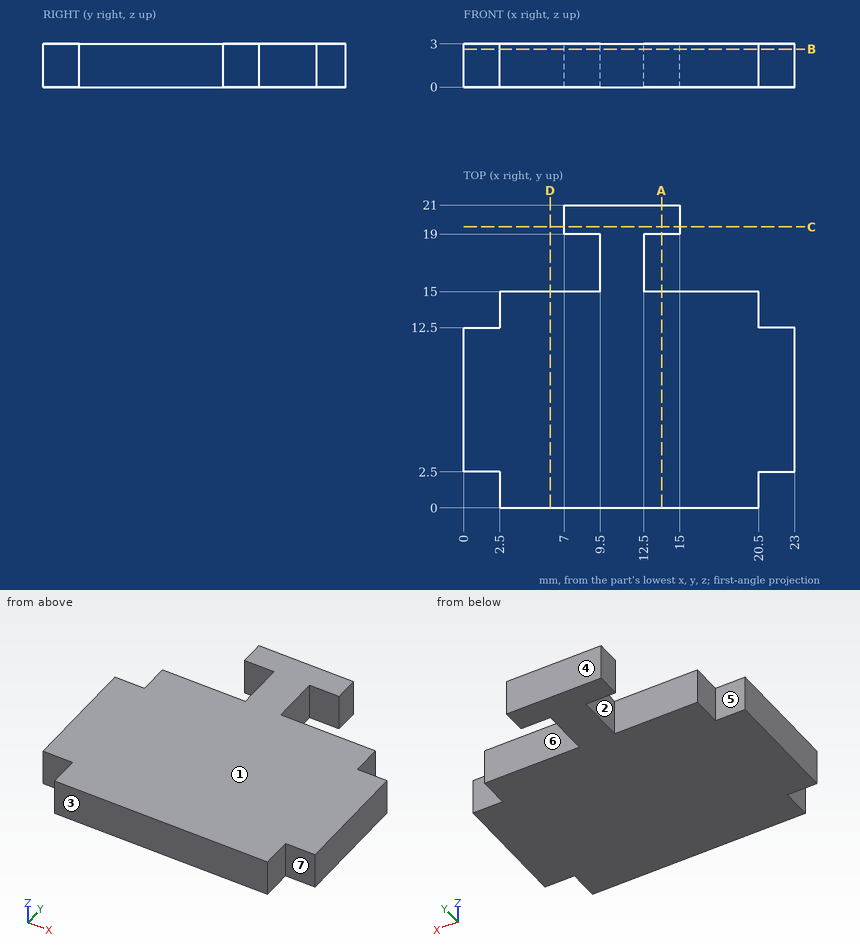
Source: three-view drawing plus pictorial views. Frame: mm from the lowest corner of the part. A direction names the side the tool comes from. Round coordinates to 2 decimals unless told otherwise and drop trailing zeros. Loops run counter-clockwise (first coordinate to the right, second up) from the corner with the lowest first, then second, coordinate; pieces in that order, holes last. Notation, with made-up numbers: M 59,72.25 L 64,72.25 A24 cw 64,87.25 Z; hole C 60.25,20 d1. An arc over 180 degrees is marked long. Answer as CSV lines item,"result". Start each with the question number.
(1) Section A-A, the plane x = 13.75. Output: boundary loops of the cut face in (y, z).
(2) Section D-D, the plane x = 6. Output: boundary loops of the cut face in (y, z), plus the area to 3 significant figures.
(3) First-contact query: pin 1 (1 mm diameter, centred on y = 20, z = 2, fed in from +X); pin 2 (0.8 mm diameter, centred on y = 13.5, z = 1.5, fed in from +X); pin 3 (1.5 mm diameter, centred on y = 17.5, z = 1, fed in from -X). Flat tips, straight axial feed; report the tip coordinate or a pass-through.
(4) Section C-C, the plane y = 19.5. Output: boundary loops of the cut face in (x, z), plus the area to 3 significant figures.
(5) Line query: line 1 (Y direction, x = 9, z = 1.7); line 2 (Y direction, x = 6.75, z = 2.2); line 3 (X direction, y = 17, z = 0.25). Output: solid intervals per line, ascending. Write a range as [from, to].
(6) Section B-B, the plane z = 2.65. Output: boundary loops of the cut face in (x, y), plus the area to 3 significant figures.
(7) Reachability of the marked faces 5, 6 and 7 from +Z, -Z, +X, -X, +Y, -Y: full face, straight path, thin tool, end or side. Return the list, or none.
(8) Draft query along Y for the marked faces 1, 2, 3 and 4. Return one class per face: released by +Y, released by -Y, zero draft, split by the parting line, or undercut.
Values found:
1,outline,"M 0,0 L 15,0 L 15,3 L 0,3 Z; M 19,0 L 21,0 L 21,3 L 19,3 Z"
2,outline,"M 0,0 L 15,0 L 15,3 L 0,3 Z"
2,area,"45.0 mm²"
3,pin 1,"stops at x = 15"
3,pin 2,"stops at x = 20.5"
3,pin 3,"stops at x = 9.5"
4,outline,"M 7,0 L 15,0 L 15,3 L 7,3 Z"
4,area,"24.0 mm²"
5,line 1,"y = [0, 15], [19, 21]"
5,line 2,"y = [0, 15]"
5,line 3,"x = [9.5, 12.5]"
6,outline,"M 0,2.5 L 2.5,2.5 L 2.5,0 L 20.5,0 L 20.5,2.5 L 23,2.5 L 23,12.5 L 20.5,12.5 L 20.5,15 L 12.5,15 L 12.5,19 L 15,19 L 15,21 L 7,21 L 7,19 L 9.5,19 L 9.5,15 L 2.5,15 L 2.5,12.5 L 0,12.5 Z"
6,area,"348 mm²"
7,face 5,"+Z, -Z, -X, +Y"
7,face 6,"+Z, -Z, +X"
7,face 7,"+Z, -Z, +X, -Y"
8,face 1,"zero draft"
8,face 2,"undercut"
8,face 3,"released by -Y"
8,face 4,"released by +Y"
